Autodesk Inventor part; units mm, degrees
ref_plane "YZ Plane" through (0, 0, 0) normal (1, 0, 0) x (0, 1, 0)
ref_plane "XZ Plane" through (0, 0, 0) normal (0, 1, 0) x (-1, 0, 0)
ref_plane "XY Plane" through (0, 0, 0) normal (0, 0, 1) x (1, 0, 0)
sketch "Sketch1" plane through (0, 0, 0) normal (0, 0, 1) x (1, 0, 0)
  line L0 (0, 0) -> (42.926, 0)
  line L1 (42.926, 0) -> (42.926, 43.942)
  line L2 (42.926, 43.942) -> (0, 43.942)
  line L3 (0, 43.942) -> (0, 0)
  line L4 (0, 6.35) -> (42.926, 6.35)
  line L5 (15.113, 31.75) -> (27.813, 31.75)
  line L6 (27.813, 31.75) -> (27.813, 19.05)
  line L7 (27.813, 19.05) -> (15.113, 19.05)
  line L8 (15.113, 19.05) -> (15.113, 31.75)
  point P0 (21.463, 31.75)
  point P1 (21.463, 43.942)
  dimension "d0" = 43.942
  dimension "d1" = 42.926
  dimension "d2" = 12.7
  dimension "d3" = 6.35
  dimension "d4" = 12.7
extrude "Extrusion1" add sketch "Sketch1" against normal blind 19.05 contours L3 L2 L1 L4 | L5 L6 L7 L8
extrude "Extrusion2" add sketch "Sketch1" against normal blind 32.004 contours L3 L4 L1 L0
extrude "Extrusion3" add sketch "Sketch1" along normal blind 1.27 contours L5 L6 L7 L8
sketch "Sketch2" plane through (0, 6.35, -19.05) normal (0, 1, 0) x (1, 0, 0)
  line L0 (0, 0) -> (0, 12.954)
  line L1 (42.926, 0) -> (42.926, 12.954)
  point P0 (0, -19.05)
  point P1 (35.306, 6.477)
  point P2 (7.62, 6.477)
  point P3 (0, 6.477)
  dimension "d11" = 7.62
  dimension "d12" = 7.62
hole "Hole1" at (35.306, 6.35, -25.527) at (7.62, 6.35, -25.527) direction (0, -1, 0) diameter 3.81 end through all
fillet "Fillet1" radius 3.175 2 edges at (42.926, 3.175, -32.004) (0, 3.175, -32.004)
properties part number "OGLiDAR" material "LCP Plastic"
The model under review builds one solid part; all positions refer to its coordinate system, in mm. A direction names the side the tool comes from. Coordinates: 2 decimals unless noted, no trailing zeros. Write each loop counter-clockwise with the first axis right and the second up, starting at its lowest first coordinate (ties: lowest second). Pieces come first, ordered by that corner, then holes. Notation, with made-up numbers: (51, -21.75) - (83, -21.75) arc R24 cw to (83, 7.25) - close; hole circle Ø7 at (61, 24). An arc over 180 degrees is marked (long way). Answer as CSV lines item,"result".
(1) Mouldability with a two-part tool opening along Z and no side actions: class faces 4 (the flat face through (21, 25, 1.27)), 5 (the cylindrical face through (42.02, 3.22, -31.05)), 6 (the cylindrical face through (37.166, 3.131, -25.94)), 7 (the flat face through (0, 22, -11)) as pulls with the +Z half, pulls with the -Z half, needs draft (parallel to the pull), parting line crosses it, or undercut.
Data:
face 4,"pulls with the +Z half"
face 5,"pulls with the -Z half"
face 6,"undercut"
face 7,"needs draft"
(2) Clearance check with flat-ended pins moving along their axes: pin 1 Ø1 at (x, y) = (17, 32.5) entering from -Z; pin 2 Ø5 at (y, z) = (12, -22.5) entering from +X; pin 3 Ø3 at (x, y) = (37, 23) entering from +Z; pin 4 Ø4 at (x, z) = (16, -23.5) entering from +Y. State where each tip first meets the part, or that it passes through.
Data:
pin 1,"stops at z = -19.05"
pin 2,"passes through"
pin 3,"stops at z = 0"
pin 4,"stops at y = 6.35"
(3) We need section A-A (x = 7.62). Give the boundary of the cut face in (y, z).
Data:
outline,"(0, -32) - (6.35, -32) - (6.35, -27.43) - (0, -27.43) - close; (0, -23.62) - (6.35, -23.62) - (6.35, -19.05) - (43.94, -19.05) - (43.94, 0) - (0, 0) - close"
(4) For line 1 along Z through (x, y) = (7.62, 3.5); line 2 along Y through (x, z) = (2.5, -26); line 3 along Z through (x, y) = (38, 11), list the stretches that pass through material, from the lowest coordinate up. Write a range as [from, to].
Data:
line 1,"z = [-32, -27.43], [-23.62, 0]"
line 2,"y = [0, 6.35]"
line 3,"z = [-19.05, 0]"
(5) We need section C-C (y = 8). Give the boundary of the cut face in (x, z), plus the area to 3 significant figures.
Data:
outline,"(0, -19.05) - (42.93, -19.05) - (42.93, 0) - (0, 0) - close"
area,"818 mm2"
(6) We need section D-D (x = 36.5). Give the boundary of the cut face in (y, z).
Data:
outline,"(0, -32) - (6.35, -32) - (6.35, -27.01) - (0, -27.01) - close; (0, -24.04) - (6.35, -24.04) - (6.35, -19.05) - (43.94, -19.05) - (43.94, 0) - (0, 0) - close"
(7) Tool access review of faces 1 (the flat face through (22, 19.05, 1)), 2 (the flat face through (21, 31.75, 1)), 3 (the flat face through (21, 6.35, -25)): name each direction out of +Z, -Z, +X, -X, +Y, -Y from which nothing blocks a thin tool from reaching the whole face with its end or side.
Data:
face 1,"+Z, +X, -X, -Y"
face 2,"+Z, +X, -X, +Y"
face 3,"-Z, +X, -X, +Y"
(8) We need section B-B (x = 26.5). Give the boundary of the cut face in (y, z), plus the area to 3 significant figures.
Data:
outline,"(0, -32) - (6.35, -32) - (6.35, -19.05) - (43.94, -19.05) - (43.94, 0) - (31.75, 0) - (31.75, 1.27) - (19.05, 1.27) - (19.05, 0) - (0, 0) - close"
area,"935 mm2"
